CAD build for the part. Positions are in the model's coordinates, mm. A direction names the side the tool comes from. Give positions to 0.01 mm unless a question says otherwise; leave off trailing zeros. Write each loop counter-clockwise with the first axis right and the second up, starting at its lowest first coordinate (ties: lowest second). Pieces come first, ordered by that corner, then holes. Notation, with made-up numbers: (-16, 19) -> (-11, 19) arc R30 cw to (-11, 50) -> close; hole circle Ø9 at (35.5, -38). An arc over 180 degrees is marked (long way). Answer in a Markdown table with one row per item. Add a question column.
```python
from build123d import *

# Parameters (mm, degrees)
F2_R     = 4.7625
F3_DEPTH = 9.525
F4_R     = 1.5875
F5_DEPTH = 22.225


with BuildPart() as f1:
    # F0 (on Front) → F1 (revolve)
    with BuildSketch(Plane.XZ):
        Polygon((0, 48.946209), (0, 0), (26.086207, 20.739919), (26.086207, 30.510725), (13.734438, 30.510725), (9.678629, 36.410082), (9.678629, 48.946209), align=None)
    revolve(axis=Axis((0, 0, 24.473105), (0, 0, -1)))

    # F2 (on face) → F3 (cut)
    with BuildSketch(Plane.XY.offset(48.946209)):
        Circle(F2_R)
    extrude(amount=-F3_DEPTH, mode=Mode.SUBTRACT)

    # F4 (on Top) → F5 (cut)
    with BuildSketch(Plane.XY):
        Circle(F4_R)
    extrude(amount=F5_DEPTH, mode=Mode.SUBTRACT)


solid = f1.part
```
Item 1: Mould opens along X. For faces 3 (the face through (0, 0, 22.225)), 4 (the face through (-20.701, 15.873, 25.694)), 5 (the face through (-4.4, -2.3, 48.946)) say: released by +X, released by -X, zero draft, split by the parting line, or undercut.
Item 2: Which spindle directions (+Z, -Z, +X, -X, +Y, -Y) get a long thin tool onto all of the face, cutting with end or side? Do faces 1 (the face through (-3.78, -2.9, 44.25)), 2 (the face through (-0.34, -1.55, 11.6)). Say none if no direction does.
Item 3: Probe L1, parallel to Y at x = 0, z = 43.5; L2, parallel to X at y = 0, z = 6; L3, parallel to Y at x = 0, z = 7. List the from-to ranges inside material, lowest first. Write a range as from..to.
Item 4: Drop flat-ended pins along their axis: pin 1 Ø3.5 at (x, y) = (0, 0) entering from -Z; pin 2 Ø5 at (x, z) = (-8, 6.5) entering from -Y; pin 3 Ø2 at (x, y) = (-13, -15) entering from -Z; pin 4 Ø2 at (y, z) = (13, 14) entering from +X. Give the stop position or say it passes through.
Item 5: Slice it at C-C, the plane z = 38. List the corners of the cut face in (x, y).
Item 6: Slice it at A-A, the plane x = 0. List the corners of the cut face in (y, z) (1 decimal), then the cut area to 3 significant figures.
Item 7: Slice it at D-D, the plane z = 43. List the corners of the cut face in (x, y) (1 decimal), then the cut area to 3 significant figures.
Answer key:
| question | item | result |
|---|---|---|
| 1 | face 3 | undercut |
| 1 | face 4 | split by the parting line |
| 1 | face 5 | zero draft |
| 2 | face 1 | +Z |
| 2 | face 2 | -Z |
| 3 | L1 | y = -9.68..-4.76, 4.76..9.68 |
| 3 | L2 | x = -7.55..-1.59, 1.59..7.55 |
| 3 | L3 | y = -8.8..-1.59, 1.59..8.8 |
| 4 | pin 1 | stops at z = 1.26 |
| 4 | pin 2 | stops at y = -8.57 |
| 4 | pin 3 | stops at z = 14.99 |
| 4 | pin 4 | stops at x = 13.91 |
| 5 | outline | circle Ø19.36 at (0, 0) |
| 6 | outline | (-26.1, 20.7) -> (-1.6, 1.3) -> (-1.6, 22.2) -> (1.6, 22.2) -> (1.6, 1.3) -> (26.1, 20.7) -> (26.1, 30.5) -> (13.7, 30.5) -> (9.7, 36.4) -> (9.7, 48.9) -> (4.8, 48.9) -> (4.8, 39.4) -> (-4.8, 39.4) -> (-4.8, 48.9) -> (-9.7, 48.9) -> (-9.7, 36.4) -> (-13.7, 30.5) -> (-26.1, 30.5) -> close |
| 6 | area | 1,270 mm² |
| 7 | outline | circle Ø19.4 at (0, 0); hole circle Ø9.5 at (0, 0) |
| 7 | area | 223 mm² |
